Autodesk Fusion 360 part; units mm, degrees
sketch "Sketch1" plane through (0, 0, 0) normal (0, 0, 1) x (1, 0, 0)
  circle A0 centre (0, 0) radius 50
  circle A1 centre (0, 40) radius 4.25
  circle A2 centre (-23.5114, 32.3607) radius 4.25
  circle A3 centre (-38.0423, 12.3607) radius 4.25
  circle A4 centre (-38.0423, -12.3607) radius 4.25
  circle A5 centre (-23.5114, -32.3607) radius 4.25
  circle A6 centre (0, -40) radius 4.25
  circle A7 centre (23.5114, -32.3607) radius 4.25
  circle A8 centre (38.0423, -12.3607) radius 4.25
  circle A9 centre (38.0423, 12.3607) radius 4.25
  circle A10 centre (23.5114, 32.3607) radius 4.25
  line L0 (-3.4339, 13.9827) -> (3.4942, 14.0175)
  line L1 (3.4942, 14.0175) -> (6.9281, 20.0348)
  line L2 (6.9281, 20.0348) -> (3.4339, 26.0173)
  line L3 (3.4339, 26.0173) -> (-3.4942, 25.9825)
  line L4 (-3.4942, 25.9825) -> (-6.9281, 19.9652)
  line L5 (-6.9281, 19.9652) -> (-3.4339, 13.9827)
  line L6 (-20.7544, 3.9827) -> (-13.8263, 4.0175)
  line L7 (-13.8263, 4.0175) -> (-10.3924, 10.0348)
  line L8 (-10.3924, 10.0348) -> (-13.8866, 16.0173)
  line L9 (-13.8866, 16.0173) -> (-20.8147, 15.9825)
  line L10 (-24.2486, 9.9652) -> (-20.7544, 3.9827)
  line L11 (-20.8147, 15.9825) -> (-24.2486, 9.9652)
  line L12 (-13.8263, -15.9825) -> (-10.3924, -9.9652)
  line L13 (-10.3924, -9.9652) -> (-13.8866, -3.9827)
  line L14 (-13.8866, -3.9827) -> (-20.8147, -4.0175)
  line L15 (-20.8147, -4.0175) -> (-24.2486, -10.0348)
  line L16 (-20.7544, -16.0173) -> (-13.8263, -15.9825)
  line L17 (-24.2486, -10.0348) -> (-20.7544, -16.0173)
  line L18 (6.9281, -19.9652) -> (3.4339, -13.9827)
  line L19 (3.4339, -13.9827) -> (-3.4942, -14.0175)
  line L20 (-3.4942, -14.0175) -> (-6.9281, -20.0348)
  line L21 (-6.9281, -20.0348) -> (-3.4339, -26.0173)
  line L22 (3.4942, -25.9825) -> (6.9281, -19.9652)
  line L23 (-3.4339, -26.0173) -> (3.4942, -25.9825)
  line L24 (20.7544, -3.9827) -> (13.8263, -4.0175)
  line L25 (13.8263, -4.0175) -> (10.3924, -10.0348)
  line L26 (10.3924, -10.0348) -> (13.8866, -16.0173)
  line L27 (13.8866, -16.0173) -> (20.8147, -15.9825)
  line L28 (24.2486, -9.9652) -> (20.7544, -3.9827)
  line L29 (20.8147, -15.9825) -> (24.2486, -9.9652)
  line L30 (13.8263, 15.9825) -> (10.3924, 9.9652)
  line L31 (10.3924, 9.9652) -> (13.8866, 3.9827)
  line L32 (13.8866, 3.9827) -> (20.8147, 4.0175)
  line L33 (20.8147, 4.0175) -> (24.2486, 10.0348)
  line L34 (20.7544, 16.0173) -> (13.8263, 15.9825)
  line L35 (24.2486, 10.0348) -> (20.7544, 16.0173)
  circle A11 centre (0, 0) radius 6
  point P0 (0, 20)
  dimension "d3" = 100
  dimension "d4" = 8.5
  dimension "d5" = 40
  dimension "d7" = 360
  dimension "d9" = 6
  dimension "d10" = 20
  dimension "d12" = 360
  dimension "d16" = 12
extrude "Extrude1" add sketch "Sketch1" along normal blind 20 contours A0 | A11 makes body 1
copy_body "Body->Comp1" bodies 1 removing the originals makes body 2 in component "Component"
extrude "Extrude1'" cut sketch "Sketch1" along normal blind 21.019 contours A11 bodies 2 in component "Component"
component "Component" placed x (1, 0, 0) y (0, 1, 0) z (0, 0, 1) at (0, 0, 0)
equation "Reaktion_Durchmesser = 120 mm"
equation "M8_Durchmesser = 8.5 mm"
equation "d4 = M8_Durchmesser"
equation "Plygon_D = 6 mm"
equation "wheel_hohe = 20 mm"
equation "d14 = wheel_hohe"
Source: CAD feature listing. Evaluate the final solid. Frame: model axes, mm. Coordinates: 2 decimals unless noted, no trailing zeros. Order: outer loops, then holes, each group sorted by start corner. A loop starts at its lowest first (then second) coordinate and runs counter-clockwise, first axis right, second up.
Item 1: Pull-direction query (Y, two-part tool) for faces 1 (the face through (12.115, 7.016, 9.86)), 2 (the face through (10, 1, 0)), 3 (the face through (47.69, -15.02, 9.86)); classes: pulls with the +Y half, pulls with the -Y half, needs draft (parallel to the pull), parting line crosses it, or undercut.
Output values:
face 1: undercut
face 2: needs draft
face 3: parting line crosses it
Item 2: Material intervals for line 1 (Y direction, x = 0, z = 12.5); line 2 (Y direction, x = 40, z = 14); line 3 (Y direction, x = -40.5, z = 3), sorted ascending.
Output values:
line 1: y = -50 to -44.25, -35.75 to -26, -14 to -6, 6 to 14, 26 to 35.75, 44.25 to 50
line 2: y = -30 to -16.13, -8.59 to 8.59, 16.13 to 30
line 3: y = -29.32 to -15.83, -8.89 to 8.89, 15.83 to 29.32
Item 3: Cut plane A-A (y = 40). Return loops of the section in (x, z).
Output values:
outline: (-30, 0) - (-4.25, 0) - (-4.25, 20) - (-30, 20) - close; (4.25, 0) - (30, 0) - (30, 20) - (4.25, 20) - close
Item 4: First-contact query: P1, Ø2, axis at y = 3.5, z = 2, coming from the +X side; P2, Ø8, axis at x = 32, z = 17, coming from the +Y side; P3, Ø3, axis at x = 26, z = 11.5, coming from the -Y side. Flat tips, straight axial feed; report the tip coordinate or a pass-through.
Output values:
P1: stops at x = 49.94
P2: stops at y = 41.42
P3: stops at y = -43.59
Item 5: Cut plane B-B (x = 2). Return loops of the section in (y, z).
Output values:
outline: (-49.96, 0) - (-43.75, 0) - (-43.75, 20) - (-49.96, 20) - close; (-36.25, 0) - (-25.99, 0) - (-25.99, 20) - (-36.25, 20) - close; (-13.99, 0) - (-5.66, 0) - (-5.66, 20) - (-13.99, 20) - close; (5.66, 0) - (14.01, 0) - (14.01, 20) - (5.66, 20) - close; (26.01, 0) - (36.25, 0) - (36.25, 20) - (26.01, 20) - close; (43.75, 0) - (49.96, 0) - (49.96, 20) - (43.75, 20) - close
Item 6: Cut plane D-D (z = 10.75). Count the separate pieces of the cut face and the enclosed holes in it, plus the area to 3 significant figures.
Output values:
separate pieces: 1
enclosed holes: 17
area: 6,430 mm2
Item 7: Cut plane C-C (y = 0). Return loops of the section in (x, z).
Output values:
outline: (-50, 0) - (-6, 0) - (-6, 20) - (-50, 20) - close; (6, 0) - (50, 0) - (50, 20) - (6, 20) - close
